Can you work these out from the model? Positions are in its coordinate system, mm. Face numbers are marked on the shaded views. A direction names the side the tool comes from. Round coordinates to 2 decimals unless told otherwise and drop trailing zeros. Order: outer loops, then holes, each group sorted by start corner. A loop starts at its lowest first (then second) coordinate and runs counter-clockwise, first axis right, second up. Notation, with made-up numbers: M -29.75,76 L -13.75,76 A24 ccw -13.75,88 Z; hole C -4,-21.75 d7. An arc over 180 degrees is marked long. Answer as CSV lines item,"result". Start each with the question number.
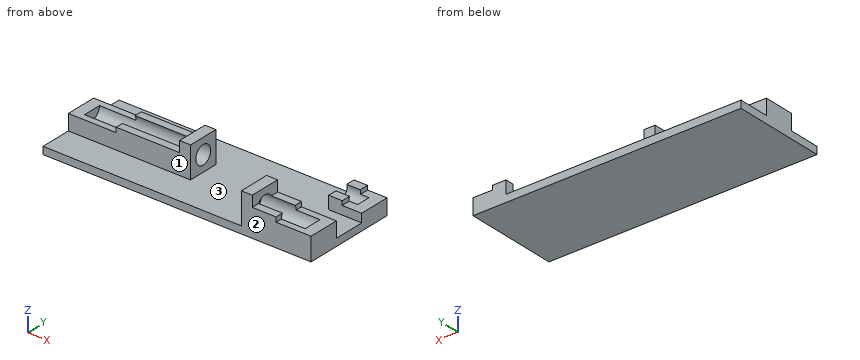
from build123d import *

# Parameters (mm, degrees)
CROQUIS1_W              = 73
CROQUIS1_H              = 25.5
SALIENTE_EXTRUIR1_DEPTH = 2
CROQUIS2_W              = 3
CROQUIS2_H              = 8.5
SALIENTE_EXTRUIR2_DEPTH = 8.5
CROQUIS4_W              = 13
CROQUIS4_H              = 8.5
CROQUIS4_W_2            = 27.3
SALIENTE_EXTRUIR3_DEPTH = 6.05
CORTAR_EXTRUIR1_START   = -16
CROQUIS5_R              = 2.5
CORTAR_EXTRUIR1_DEPTH   = 16
CORTAR_EXTRUIR2_START   = -30.3
CROQUIS6_R              = 2.5
CORTAR_EXTRUIR2_DEPTH   = 30.3
CROQUIS7_W              = 10
CROQUIS7_H              = 8.5
CROQUIS7_W_2            = 6.5
CORTAR_EXTRUIR3_DEPTH   = 1.8
CROQUIS8_W              = 3
CROQUIS8_H              = 8.5
SALIENTE_EXTRUIR4_DEPTH = 4.85
CROQUIS9_R              = 1.95
CORTAR_EXTRUIR4_DEPTH   = 6
CORTAR_EXTRUIR5_START   = -3.65
CROQUIS10_W             = 3
CROQUIS10_H             = 8.5
CORTAR_EXTRUIR5_DEPTH   = 3.65
CORTAR_EXTRUIR6_START   = -4.25
CROQUIS11_W             = 3
CROQUIS11_H             = 8.5
CORTAR_EXTRUIR6_DEPTH   = 4.25
CROQUIS12_W             = 17.3
CROQUIS12_H             = 8.5
CROQUIS12_W_2           = 6.5
CORTAR_EXTRUIR7_DEPTH   = 0.5
CROQUIS13_W             = 5.3
CROQUIS13_H             = 8.5
CORTAR_EXTRUIR8_DEPTH   = 2.5
CROQUIS15_W             = 4.5
CROQUIS15_H             = 8.5
CORTAR_EXTRUIR9_DEPTH   = 5


with BuildPart() as part:
    # Croquis1 → Saliente-Extruir1 (new body)
    with BuildSketch(Plane.XY):
        with Locations((-50.046391753, 8.196735395)):
            Rectangle(CROQUIS1_W, CROQUIS1_H)
    extrude(amount=SALIENTE_EXTRUIR1_DEPTH)

    # Croquis2 → Saliente-Extruir2 (add)
    with BuildSketch(Plane.XY.offset(2)):
        with Locations((-15.046391753, 16.696735395)):
            Rectangle(CROQUIS2_W, CROQUIS2_H)
        with Locations((-15.046391753, -0.303264605)):
            Rectangle(CROQUIS2_W, CROQUIS2_H)
        with Locations((-85.046391753, 8.196735395)):
            Rectangle(CROQUIS2_W, CROQUIS2_H)
        with Locations((-21.046391753, 16.696735395)):
            Rectangle(CROQUIS2_W, CROQUIS2_H)
        with Locations((-31.046391753, -0.303264605)):
            Rectangle(CROQUIS2_W, CROQUIS2_H)
        with Locations((-54.746391753, 8.196735395)):
            Rectangle(CROQUIS2_W, CROQUIS2_H)
    extrude(amount=SALIENTE_EXTRUIR2_DEPTH)

    # Croquis4 → Saliente-Extruir3 (add)
    with BuildSketch(Plane.XY.offset(2)):
        with Locations((-23.046391753, -0.303264605)):
            Rectangle(CROQUIS4_W, CROQUIS4_H)
        with Locations((-69.896391753, 8.196735395)):
            Rectangle(CROQUIS4_W_2, CROQUIS4_H)
    extrude(amount=SALIENTE_EXTRUIR3_DEPTH)

    # Croquis5 → Cortar-Extruir1 (cut)
    with BuildSketch(Plane.ZY.offset(32.546391753).offset(CORTAR_EXTRUIR1_START)):
        with Locations((6.25, -0.303264605)):
            Circle(CROQUIS5_R)
    extrude(amount=CORTAR_EXTRUIR1_DEPTH, mode=Mode.SUBTRACT)

    # Croquis6 → Cortar-Extruir2 (cut)
    with BuildSketch(Plane(origin=(-53.246391753, 0, 0), x_dir=(0, 0, -1), z_dir=(1, 0, 0)).offset(CORTAR_EXTRUIR2_START)):
        with Locations((-6.25, 8.196735395)):
            Circle(CROQUIS6_R)
    extrude(amount=CORTAR_EXTRUIR2_DEPTH, mode=Mode.SUBTRACT)

    # Croquis7 → Cortar-Extruir3 (cut)
    with BuildSketch(Plane.XY.offset(8.05)):
        with Locations((-78.546391753, 8.196735395)):
            Rectangle(CROQUIS7_W, CROQUIS7_H)
        with Locations((-19.796391753, -0.303264605)):
            Rectangle(CROQUIS7_W_2, CROQUIS7_H)
    extrude(amount=-CORTAR_EXTRUIR3_DEPTH, mode=Mode.SUBTRACT)

    # Croquis8 → Saliente-Extruir4 (add)
    with BuildSketch(Plane.XY.offset(2)):
        with Locations((-18.046391753, 16.696735395)):
            Rectangle(CROQUIS8_W, CROQUIS8_H)
    extrude(amount=SALIENTE_EXTRUIR4_DEPTH)

    # Croquis9 → Cortar-Extruir4 (cut)
    with BuildSketch(Plane.ZY.offset(22.546391753)):
        with Locations((4.75, 16.696735395)):
            Circle(CROQUIS9_R)
    extrude(amount=-CORTAR_EXTRUIR4_DEPTH, mode=Mode.SUBTRACT)

    # Croquis10 → Cortar-Extruir5 (cut)
    with BuildSketch(Plane.XY.offset(10.5).offset(CORTAR_EXTRUIR5_START)):
        with Locations((-15.046391753, 16.696735395)):
            Rectangle(CROQUIS10_W, CROQUIS10_H)
    extrude(amount=CORTAR_EXTRUIR5_DEPTH, mode=Mode.SUBTRACT)

    # Croquis11 → Cortar-Extruir6 (cut)
    with BuildSketch(Plane.XY.offset(10.5).offset(CORTAR_EXTRUIR6_START)):
        with Locations((-15.046391753, -0.303264605)):
            Rectangle(CROQUIS11_W, CROQUIS11_H)
        with Locations((-85.046391753, 8.196735395)):
            Rectangle(CROQUIS11_W, CROQUIS11_H)
    extrude(amount=CORTAR_EXTRUIR6_DEPTH, mode=Mode.SUBTRACT)

    # Croquis12 → Cortar-Extruir7 (cut)
    with BuildSketch(Plane.XY.offset(8.05)):
        with Locations((-64.896391753, 8.196735395)):
            Rectangle(CROQUIS12_W, CROQUIS12_H)
        with Locations((-26.296391753, -0.303264605)):
            Rectangle(CROQUIS12_W_2, CROQUIS12_H)
    extrude(amount=-CORTAR_EXTRUIR7_DEPTH, mode=Mode.SUBTRACT)

    # Croquis13 → Cortar-Extruir8 (cut)
    with BuildSketch(Plane.XY.offset(6.85)):
        with Locations((-16.196391753, 16.696735395)):
            Rectangle(CROQUIS13_W, CROQUIS13_H)
    extrude(amount=-CORTAR_EXTRUIR8_DEPTH, mode=Mode.SUBTRACT)

    # Croquis15 → Cortar-Extruir9 (cut)
    with BuildSketch(Plane.XY.offset(10.5)):
        with Locations((-20.296391753, 16.696735395)):
            Rectangle(CROQUIS15_W, CROQUIS15_H)
    extrude(amount=-CORTAR_EXTRUIR9_DEPTH, mode=Mode.SUBTRACT)


solid = part.part
(1) I'm going to push flat-ended pins straight in: P1, Ø2.5, axis at y = 1, z = 6, coming from the -X side; P2, Ø0.6, axis at y = 20, z = 5, coming from the +X side; P3, Ø2, axis at x = -20, y = 14, coming from the +Z side. Where does each tip first touch, or does it pass through?
(2) For the marked faces 1, 2 and 3, which set-ups out of +Z, -Z, +X, -X, +Y, -Y let a thin tool reach every point of the face, with its end or its side?
(3) I want a section at A-A on x = -71. Write out the boundary of the cut face in (y, z), and give its area (3 significant figures).
(4) I want a section at B-B on y = 9.5. Write out the boundary of the cut face in (x, z).
(5) I want a section at C-C on x = -45. Write out the boundary of the cut face in (y, z).
(6) If I drill on line 1 along Y through (x, z) = (-67, 6.25); line 2 along Y through (x, z) = (-23.5, 6.25); line 3 along Y through (x, z) = (-19.15, 4.75), over which ranges is the centre line in solid material (lowest first)?
From the geometry:
1,P1,"x = -32.55"
1,P2,"x = -18.85"
1,P3,"z = 5.5"
2,face 1,"+Z, -X, -Y"
2,face 2,"+Z, -Z, +X, -X, -Y"
2,face 3,"+Z"
3,outline,"M -4.55,0 L 20.95,0 L 20.95,2 L 12.45,2 L 12.45,7.55 L 10.33,7.55 A2.5 cw long 6.06,7.55 L 3.95,7.55 L 3.95,2 L -4.55,2 Z"
3,area,"82.2 mm²"
4,outline,"M -86.55,0 L -13.55,0 L -13.55,2 L -53.25,2 L -53.25,4.12 L -83.55,4.12 L -83.55,6.25 L -86.55,6.25 Z; M -56.25,8.38 L -53.25,8.38 L -53.25,10.5 L -56.25,10.5 Z"
5,outline,"M -4.55,0 L 20.95,0 L 20.95,2 L -4.55,2 Z"
6,line 1,"3.95 to 5.7, 10.7 to 12.45"
6,line 2,"-4.55 to -2.8, 2.2 to 3.95"
6,line 3,"-4.55 to -2.3, 1.7 to 3.95, 12.45 to 14.75, 18.65 to 20.95"
